The listing builds one solid part. Answer for the finished solid, in the listing's coordinates (mm). Give positions to 0.01 mm unless a question says otherwise; leave off trailing zeros. Order: outer loops, then holes, each group sorted by start corner. A loop starts at its lowest first (then second) coordinate and runs counter-clockwise, first axis right, second up. Notation, with made-up numbers: M 36.25,55 L 81.25,55 A23 cw 81.25,68 Z; hole C -5.5,-35 d1. An arc over 180 degrees is marked long. Answer as a JSON object with one key per item and string values. Group by question number.
Autodesk Inventor part; units mm, degrees
ref_plane "YZ Plane" through (0, 0, 0) normal (1, 0, 0) x (0, 1, 0)
ref_plane "XZ Plane" through (0, 0, 0) normal (0, 1, 0) x (-1, 0, 0)
ref_plane "XY Plane" through (0, 0, 0) normal (0, 0, 1) x (1, 0, 0)
sketch "Sketch1" plane through (0, 0, 0) normal (0, 0, 1) x (1, 0, 0)
  line L0 (-70.3712, 150.7033) -> (79.6288, 150.7033)
  line L1 (79.6288, 150.7033) -> (79.6288, -149.2967)
  line L2 (79.6288, -149.2967) -> (-70.3712, -149.2967)
  line L3 (-70.3712, -149.2967) -> (-70.3712, 150.7033)
  point P0 (0, 0)
extrude "Extrusion1" add sketch "Sketch1" along normal blind 3
sketch "Sketch2" plane through (0, 0, 3) normal (0, 0, 1) x (1, 0, 0)
  line L0 (-70.3712, 150.7033) -> (-70.3712, -149.2967)
  line L1 (-70.3712, 271.0495) -> (-120.3712, 271.0495)
  line L2 (-20.3712, 147.7184) -> (-20.3712, 150.7184)
  line L3 (-20.3712, 147.7184) -> (29.6288, 147.7184)
  line L4 (29.6288, 147.7184) -> (29.6288, 150.7184)
  line L5 (-20.3712, 150.7184) -> (29.6288, 150.7184)
  line L6 (79.6288, 150.7033) -> (-70.3712, 150.7033)
  point P0 (0, 0)
  dimension "d9" = 50
extrude "Extrusion2" cut sketch "Sketch2" against normal blind 3
sketch "Sketch3" plane through (0, 0, 3) normal (0, 0, 1) x (1, 0, 0)
  line L0 (-20.3712, 150.7033) -> (-20.3712, 147.7184)
  line L1 (-20.3712, -149.2722) -> (29.6288, -149.2967)
  line L2 (79.6288, -149.2967) -> (-70.3712, -149.2967)
  line L3 (-20.3712, -149.2722) -> (-20.3712, -146.2722)
  line L4 (-20.3712, -146.2722) -> (29.6288, -146.2967)
  line L5 (29.6288, -146.2967) -> (29.6288, -149.2967)
  point P0 (0, 0)
extrude "Extrusion3" cut sketch "Sketch3" against normal blind 3
sketch "Sketch4" plane through (0, 0, 3) normal (0, 0, 1) x (1, 0, 0)
  line L0 (29.6288, -46.2722) -> (-20.3712, -46.2722)
  line L1 (-20.3712, -46.2722) -> (29.6288, -46.2722)
  line L2 (29.6288, -46.2722) -> (29.6288, -43.6172)
  line L3 (29.6288, -43.6172) -> (-20.3712, -43.6172)
  line L4 (-20.3712, -43.6172) -> (-20.3712, -46.2722)
  point P0 (0, 0)
extrude "Extrusion4" add sketch "Sketch4" against normal blind 3
sketch "Sketch5" plane through (0, 0, 3) normal (0, 0, 1) x (1, 0, 0)
  line L0 (-20.3712, -42.9205) -> (29.6288, -42.9205)
  line L1 (29.6288, -42.9205) -> (29.6288, -39.9205)
  line L2 (29.6288, -39.9205) -> (-20.3712, -39.9205)
  line L3 (-20.3712, -39.9205) -> (-20.3712, -42.9205)
  point P0 (0, 0)
  point P1 (-20.3712, -146.2722)
  point P2 (29.6288, -146.2967)
extrude "Extrusion5" cut sketch "Sketch5" against normal blind 3
sketch "Sketch6" plane through (0, 0, 3) normal (0, 0, 1) x (1, 0, 0)
  line L0 (29.6288, -39.9205) -> (-20.3712, -39.9205)
  line L1 (-20.3712, 60.1524) -> (29.6288, 60.1524)
  line L2 (29.6288, 60.1524) -> (29.6288, 63.1524)
  line L3 (29.6288, 63.1524) -> (-20.3712, 63.1524)
  line L4 (-20.3712, 63.1524) -> (-20.3712, 60.1524)
  point P0 (0, 0)
extrude "Extrusion6" cut sketch "Sketch6" against normal blind 3
sketch "Sketch7" plane through (0, 0, 3) normal (0, 0, 1) x (1, 0, 0)
  line L0 (29.6288, -149.2967) -> (-70.3712, -149.2967)
  line L1 (-70.3712, -149.2967) -> (-70.3712, 150.7033)
  circle A0 centre (4.6288, -99.2967) radius 12
  point P0 (0, 0)
extrude "Extrusion7" cut sketch "Sketch7" against normal blind 3
sketch "Sketch8" plane through (0, 0, 3) normal (0, 0, 1) x (1, 0, 0)
  circle A0 centre (4.6288, -99.2967) radius 12
  circle A1 centre (20.6853, -83.2968) radius 1.5
  circle A2 centre (-11.3147, -83.2968) radius 1.5
  circle A3 centre (-11.3712, -115.2967) radius 1.5
  circle A4 centre (20.6288, -115.2967) radius 1.5
  point P0 (0, 0)
extrude "Extrusion8" cut sketch "Sketch8" against normal blind 3 contours A1 | A2 | A3 | A4
sketch "Sketch9" plane through (0, 0, 3) normal (0, 0, 1) x (1, 0, 0)
  point P0 (0, 0)
sketch "Sketch11" plane through (0, 0, 3) normal (0, 0, 1) x (1, 0, 0)
  line L0 (-70.3712, 150.7033) -> (-70.3712, -149.2967)
  line L1 (79.6288, -149.2967) -> (79.6288, 150.7033)
  line L2 (29.6288, 60.1524) -> (-20.3712, 60.1524)
  line L3 (-20.3712, -39.9205) -> (29.6288, -39.9205)
  circle A0 centre (52.2007, 33.6284) radius 2
  circle A1 centre (52.2018, -13.1716) radius 2
  circle A2 centre (-33.7993, 33.6284) radius 2
  circle A3 centre (-33.7993, -13.1716) radius 2
  line L4 (-43.8689, 25.3776) -> (-36.8689, 25.3776)
  line L5 (-36.8689, 25.3776) -> (-36.8689, -5.0217)
  line L6 (-36.8689, -5.0217) -> (-43.8689, -5.0217)
  line L7 (-43.8689, -5.0217) -> (-43.8689, 25.3776)
  circle A4 centre (41.9518, 10.2284) radius 7
  line L8 (29.0018, -10.3751) -> (-21.9982, -10.3751)
  line L9 (-21.9982, -10.3751) -> (-21.9982, 29.6249)
  line L10 (-21.9982, 29.6249) -> (29.0018, 29.6249)
  line L11 (29.0018, 29.6249) -> (29.0018, -10.3751)
  point P0 (0, 0)
extrude "Extrusion9" cut sketch "Sketch11" against normal blind 30
sketch "Sketch12" plane through (29.6288, -149.2967, 3) normal (0.0005, 1, 0) x (1, -0.0005, 0)
  line L0 (-100, 0) -> (0, 0)
  line L1 (-50.0015, 3) -> (0, 3)
  line L2 (0, 3) -> (0, 0)
  line L3 (0, 0) -> (-50.0015, 0)
  line L4 (-50.0015, 0) -> (-50.0015, 3)
  point P0 (-29.7019, 3)
extrude "Extrusion10" cut sketch "Sketch12" against normal blind 10
sketch "Sketch13" plane through (0, 0, 3) normal (0, 0, 1) x (1, 0, 0)
  line L0 (29.6288, -146.2967) -> (-20.3712, -146.2722)
  circle A0 centre (-11.3147, -83.2968) radius 1.5
  circle A1 centre (-11.3712, -115.2967) radius 1.5
  line L1 (-11.3712, -115.2967) -> (-11.3147, -83.2968)
  circle A2 centre (20.6853, -83.2968) radius 1.5
  line L2 (20.6853, -83.2968) -> (-11.3147, -83.2968)
  line L3 (20.6853, -115.2967) -> (20.6853, -83.2968)
  line L4 (20.6853, -115.2967) -> (-11.3712, -115.2967)
  circle A3 centre (4.6288, -99.2967) radius 12
  line L5 (4.6288, -146.2844) -> (4.6288, -131.2844)
  circle A4 centre (-11.3147, -83.2968) radius 1.5
  circle A5 centre (20.6853, -83.2968) radius 1.5
  circle A6 centre (20.6853, -115.2967) radius 1.455
  circle A7 centre (-11.3712, -115.2967) radius 1.5
  point P0 (0, 0)
  dimension "d107" = 15
  dimension "d108" = 32.0565
  dimension "d109" = 31.9999
extrude "Extrusion11" add sketch "Sketch13" against normal blind 3 contours L2 L1 A0 | A0 L1 L2 | L2 L3 A2 | A2 L3 L2 | L1 L4 A1 | A1 L4 L1 | A6 L4 L3 | L3 L4 A6
sketch "Sketch14" plane through (0, 0, 3) normal (0, 0, 1) x (1, 0, 0)
  arc A0 (21.8331, -114.4024) -> (21.8331, -116.1909) centre (20.6288, -115.2967) ccw
  circle A1 centre (20.6288, -115.2967) radius 2.2964
  point P0 (0, 0)
extrude "Extrusion12" cut sketch "Sketch14" against normal blind 3
sketch "Sketch15" plane through (0, 0, 3) normal (0, 0, 1) x (1, 0, 0)
  line L0 (17.3499, -111.5348) -> (24.4453, -111.5348)
  line L1 (24.4453, -111.5348) -> (24.4453, -120.5742)
  line L2 (24.4453, -120.5742) -> (17.3499, -120.5742)
  line L3 (17.3499, -120.5742) -> (17.3499, -111.5348)
  point P0 (0, 0)
extrude "Extrusion13" cut sketch "Sketch15" against normal blind 3
sketch "Sketch16" plane through (0, 0, 3) normal (0, 0, 1) x (1, 0, 0)
  line L0 (17.3499, -111.5348) -> (24.4453, -111.5348)
  line L1 (24.4453, -120.5742) -> (17.3499, -120.5742)
  line L2 (17.3499, -111.5348) -> (24.4453, -111.5348)
  line L3 (24.4453, -111.5348) -> (24.4453, -120.5742)
  line L4 (24.4453, -120.5742) -> (17.3499, -120.5742)
  line L5 (17.3499, -120.5742) -> (17.3499, -111.5348)
  point P0 (0, 0)
extrude "Extrusion14" add sketch "Sketch16" against normal blind 3
sketch "Sketch17" plane through (0, 0, 3) normal (0, 0, 1) x (1, 0, 0)
  circle A0 centre (4.6288, -99.2967) radius 12
  circle A1 centre (4.6288, -99.2967) radius 12
  point P0 (0, 0)
extrude "Extrusion15" add sketch "Sketch17" against normal blind 3
sketch "Sketch18" plane through (0, 0, 3) normal (0, 0, 1) x (1, 0, 0)
  line L0 (29.6288, -146.2967) -> (-20.3712, -146.2722)
  circle A0 centre (-10.8712, -109.2844) radius 1.5
  circle A1 centre (20.1288, -109.2844) radius 1.5
  circle A2 centre (20.1288, -140.2844) radius 1.5
  circle A3 centre (-10.8712, -140.2844) radius 1.5
  circle A4 centre (4.6288, -124.7844) radius 12
  point P0 (0, 0)
extrude "Extrusion16" cut sketch "Sketch18" against normal blind 35.75
sketch "Sketch19" plane through (0, 0, 3) normal (0, 0, 1) x (1, 0, 0)
  point P0 (0, 0)
properties part number "MuurL"
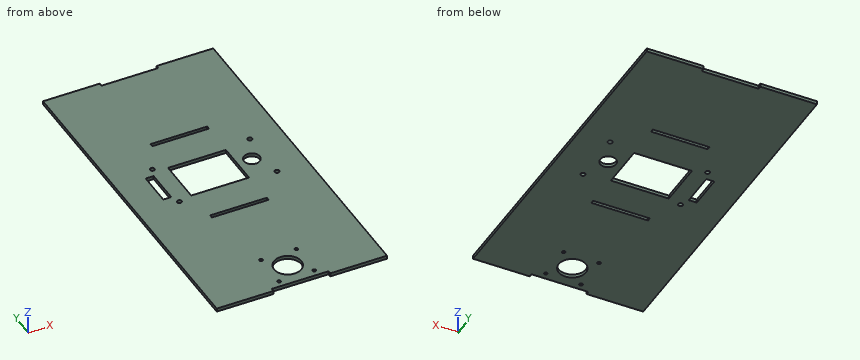
Item 1: A flat-ended cylindrical pin translates along its axis: P1, Ø0.9, axis at x = 7.5, z = 1, coming from the +Y side. Find the tip coordinate at first contact, or state that the pin passes through.
Item 2: Section D-D (z = 2) is taken. Count the separate pieces of the cut face and the enclosed holes in it, and give its area (3 significant figures).
Item 3: Section A-A (x = 13.5) is taken. Determine the outline of the cut face in (y, z).
Item 4: Consider probe 1 along Y at (x, z) = (-20, 2.25); probe 2 along Y at (x, z) = (20.5, 0.5); probe 3 along Y at (x, z) = (-38.5, 1.35). Determine where each line is inside the solid, lowest interval first. Write a range as from..to.
Item 5: Section C-C (x = -17) is taken. Determine the outline of the cut face in (y, z), and give its area (3 significant figures).
Item 6: Section B-B (x = 40.5) is taken. Determine the outline of the cut face in (y, z).
Values found:
{
 "1": {"P1": "stops at y = 147.72"},
 "2": {"separate pieces": "1", "enclosed holes": "14", "area": "41,500 mm^2"},
 "3": {"outline": "M -146.29,0 L -132.87,0 L -132.87,3 L -146.29,3 Z; M -116.7,0 L -42.92,0 L -42.92,3 L -116.7,3 Z; M -39.92,0 L -10.38,0 L -10.38,3 L -39.92,3 Z; M 29.62,0 L 60.15,0 L 60.15,3 L 29.62,3 Z; M 63.15,0 L 147.72,0 L 147.72,3 L 63.15,3 Z"},
 "4": {"probe 1": "y = -146.27..-42.92, -39.92..-10.38, 29.62..60.15, 63.15..147.72", "probe 2": "y = -146.29..-141.74, -138.83..-110.74, -107.83..-42.92, -39.92..-10.38, 29.62..60.15, 63.15..147.72", "probe 3": "y = -149.3..-5.02, 25.38..150.7"},
 "5": {"outline": "M -146.27,0 L -42.92,0 L -42.92,3 L -146.27,3 Z; M -39.92,0 L -10.38,0 L -10.38,3 L -39.92,3 Z; M 29.62,0 L 60.15,0 L 60.15,3 L 29.62,3 Z; M 63.15,0 L 147.72,0 L 147.72,3 L 63.15,3 Z", "area": "744 mm^2"},
 "6": {"outline": "M -149.3,0 L 3.38,0 L 3.38,3 L -149.3,3 Z; M 17.08,0 L 150.7,0 L 150.7,3 L 17.08,3 Z"}
}
